Build history of the part. All positions in model axes, mm. Face numbers are marked on the shaded views. Give positions to 0.01 mm unless a question says otherwise; leave off trailing zeros. Write each loop counter-clockwise with the first axis right and the second up, starting at its lowest first coordinate (ties: lowest second). Pieces come first, ordered by that corner, then holes. Notation, with made-up numbers: M 36.25,68 L 58.25,68 A19 ccw 58.25,102 Z; hole C 50,55 d9. An arc over 180 degrees is marked long. One line per item, written item: value. Start each with the question number.
Autodesk Inventor part; units mm, degrees
ref_plane "YZ Plane" through (0, 0, 0) normal (1, 0, 0) x (0, 1, 0)
ref_plane "XZ Plane" through (0, 0, 0) normal (0, 1, 0) x (-1, 0, 0)
ref_plane "XY Plane" through (0, 0, 0) normal (0, 0, 1) x (1, 0, 0)
sketch "Sketch1" plane through (0, 0, 0) normal (0, 0, 1) x (1, 0, 0)
  circle A0 centre (0, 0) radius 5.5
  dimension "d0" = 11
extrude "Extrusion1" add sketch "Sketch1" along normal blind 10
sketch "Sketch2" plane through (0, 0, 10) normal (0, 0, 1) x (1, 0, 0)
  circle A0 centre (0, 0) radius 11.15
  dimension "d3" = 22.3
extrude "Extrusion3" add sketch "Sketch2" along normal blind 38
sketch "Sketch3" plane through (0, 0, 10) normal (0, 0, -1) x (-1, 0, 0)
  circle A0 centre (0, 0) radius 10.15
  circle A1 centre (0, 0) radius 11.15
  dimension "d8" = 20.3
  dimension "d9" = 22.3
extrude "Extrusion4" add sketch "Sketch3" along normal blind 5
sketch "Sketch4" plane through (0, 0, 48) normal (0, 0, 1) x (1, 0, 0)
  circle A0 centre (0, 0) radius 14.25
  dimension "d12" = 28.5
extrude "Extrusion5" add sketch "Sketch4" along normal blind 20
fillet "Fillet1" radius 2 1 edges at (-14.25, 0, 68)
fillet "Fillet2" radius 2 1 edges at (-5.5, 0, 0)
fillet "Fillet3" radius 2 1 edges at (11.15, 0, 5)
fillet "Fillet4" radius 2 1 edges at (-14.25, 0, 48)
properties part number "Elbow_Parallel_Rod_V1"
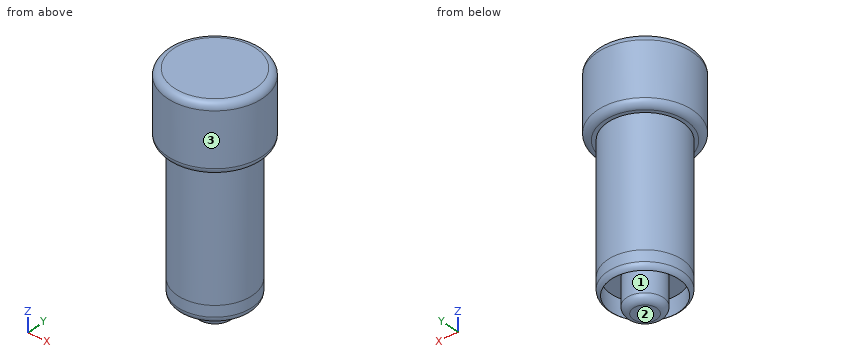
1) Band-saw the part on A-A (z = 8.5). List the corners of the cut face in (x, y).
2) Drop flat-ended pins along their axis: P1, Ø10, axis at x = -5.5, y = 8.5, coming from the -Z side; P2, Ø1, axis at y = 3.5, z = 48, coming from the -X side; P3, Ø10, axis at y = -6.5, z = 21.5, coming from the +X side. Give the stop position or say it passes through.
3) Probe line 1 along Y through (x, z) = (0, 8); line 2 along Y through (x, z) = (0, 6.05); line 3 along Z through (x, y) = (7.75, -3.75). List the from-to ranges inside material, lowest first. Write a range as from..to.
4) Mould opens along Y. For the marked faces 1, 2 and 3 say: released by +Y, released by -Y, zero draft, split by the parting line, or undercut.
5) Band-saw the part on D-D (z = 24). List the corners of the cut face in (x, y), then the cut area to 3 significant figures.
6) Band-saw the part on B-B (x = 0). List the corners of the cut face in (y, z).
Model answer:
1. outline: C 0,0 d22.3; C 0,0 d11; hole C 0,0 d20.3
2. P1: stops at z = 0.83
2. P2: stops at x = -13.13
2. P3: stops at x = 11.05
3. line 1: y = -11.15..-10.15, -5.5..5.5, 10.15..11.15
3. line 2: y = -11.03..-10.15, -5.5..5.5, 10.15..11.03
3. line 3: z = 10..68
4. face 1: undercut
4. face 2: zero draft
4. face 3: split by the parting line
5. outline: C 0,0 d22.3
5. area: 391 mm²
6. outline: M -14.25,50 A2 ccw -12.25,48 L -11.15,48 L -11.15,6.73 A2 ccw -10.15,5 L -10.15,10 L -5.5,10 L -5.5,2 A2 ccw -3.5,0 L 3.5,0 A2 ccw 5.5,2 L 5.5,10 L 10.15,10 L 10.15,5 A2 ccw 11.15,6.73 L 11.15,48 L 12.25,48 A2 ccw 14.25,50 L 14.25,66 A2 ccw 12.25,68 L -12.25,68 A2 ccw -14.25,66 Z
